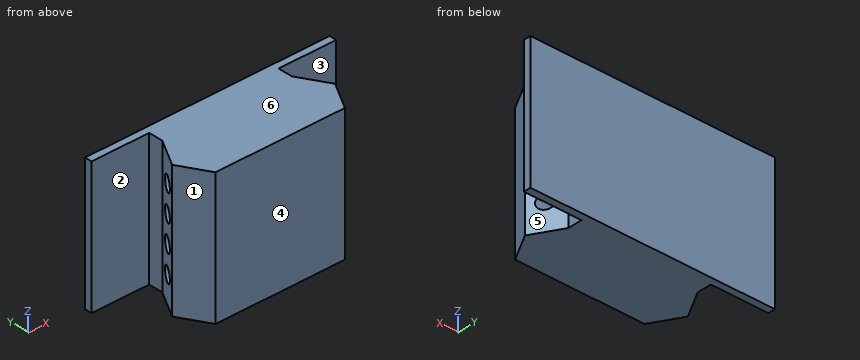
from build123d import *

# Parameters (mm, degrees)
BOSS_EXTRUDE1_DEPTH     = 18.568445
CUT_EXTRUDE1_DEPTH      = 28.942587158
CUT_EXTRUDE1_DEPTH_BACK = 28.942587158
SKETCH2_R               = 1


with BuildPart() as part:
    # Sketch1 → Boss-Extrude1 (new body)
    with BuildSketch(Plane.XY):
        Polygon((9.693000417, 0), (-8.306999583, 0), (-10.641999583, 4.044338636), (-8.306999583, 8.088677271), (-8.306999583, 10.088677271), (-16.306999583, 10.088677271), (-16.306999583, 11.088677271), (17.693000417, 11.088677271), (17.693000417, 10.088677271), (9.693000417, 10.088677271), (9.693000417, 8.088677271), (12.028000417, 4.044338636), align=None)
    extrude(amount=-BOSS_EXTRUDE1_DEPTH)

    # Sketch2 → Cut-Extrude1 (cut, two sides: drawn at the far end of the back side and taken through both)
    with BuildSketch(Plane(origin=(0, 0, 0), x_dir=(0, 0, -1), z_dir=(1, 0, 0)).offset(-CUT_EXTRUDE1_DEPTH_BACK)):
        with Locations(Location((3.71, 5.988677271, 0), (0, 0, 90))):
            Circle(SKETCH2_R)
        with Locations(Location((7.42, 5.988677271, 0), (0, 0, 90))):
            Circle(SKETCH2_R)
        with Locations(Location((11.13, 5.988677271, 0), (0, 0, 90))):
            Circle(SKETCH2_R)
        with Locations(Location((14.84, 5.988677271, 0), (0, 0, 90))):
            Circle(SKETCH2_R)
    extrude(amount=CUT_EXTRUDE1_DEPTH + CUT_EXTRUDE1_DEPTH_BACK, mode=Mode.SUBTRACT)


solid = part.part
Build history of the part. All positions in model axes, mm. Face numbers are marked on the shaded views. A direction names the side the tool comes from. Coordinates: 2 decimals unless noted, no trailing zeros. Order: outer loops, then holes, each group sorted by start corner. A loop starts at its lowest first (then second) coordinate and runs counter-clockwise, first axis right, second up. Notation, with made-up numbers: M 79.25,-39.5 L 137.25,-39.5 A19 ccw 137.25,-31.5 Z; hole C 29,75 d9. An arc over 180 degrees is marked long. One line per question, with ' | ' between items. Start each with the question number.
Q1. Flat gauge pins, fed straight in: pin 1 Ø3 at (y, z) = (5.99, -11.13) entering from -X; pin 2 Ø0.6 at (y, z) = (9.5, -5) entering from -X; pin 3 Ø6.5 at (x, z) = (-13, -10.5) entering from -Y; pin 4 Ø9 at (x, z) = (13.5, -10.5) entering from -Y. Where does each tip first touch, or does it go through?
Q2. 3-axis set-ups, long thin cutter, end or side, ignore diameter. For the marked faces 1 and 2: which of +Z, -Z, +X, -X, +Y, -Y reach the whole face in a straight line?
Q3. Saw through at A-A (y = 6.5). List the corners of the cut face in (x, z), then the cut area to 3 significant figures.
Q4. Saw through at D-D (x = -12.5). List the corners of the cut face in (y, z), then the cut area to 3 significant figures.
Q5. Probe L1, parallel to Y at x = 3, z = -11.13; L2, parallel to Z at x = 10, y = 5.25; L3, parallel to Z at x = -7, y = 5.5. List the from-to ranges inside material, lowest first. Write a range as from..to.
Q6. Saw through at B-B (x = -2). List the corners of the cut face in (y, z).
Q7. Two-plate mould, pull along Y, no slides. Class the marked faces 3, 4, 5 and 6: +Y half, -Y half, draft (parallel to the pull), parting line (faces both ways), or undercut.
Q8. Saw through at C-C (z = -7.42). List the corners of the cut face in (x, y).
Check values:
1) pin 1: stops at x = -10.38 | pin 2: stops at x = -8.31 | pin 3: stops at y = 2.5 | pin 4: stops at y = 0
2) face 1: +Z, -Z, -X, -Y | face 2: +Z, -Z, -X
3) outline: M -9.22,-18.57 L 10.61,-18.57 L 10.61,-15.7 L -9.22,-15.7 Z; M -9.22,-13.98 L 10.61,-13.98 L 10.61,-11.99 L -9.22,-11.99 Z; M -9.22,-10.27 L 10.61,-10.27 L 10.61,-8.28 L -9.22,-8.28 Z; M -9.22,-6.56 L 10.61,-6.56 L 10.61,-4.57 L -9.22,-4.57 Z; M -9.22,-2.85 L 10.61,-2.85 L 10.61,0 L -9.22,0 Z | area: 232 mm2
4) outline: M 10.09,-18.57 L 11.09,-18.57 L 11.09,0 L 10.09,0 Z | area: 18.6 mm2
5) L1: y = 0..4.99, 6.99..11.09 | L2: z = -18.57..-15.51, -14.17..-11.8, -10.46..-8.09, -6.75..-4.38, -3.04..0 | L3: z = -18.57..-15.71, -13.97..-12, -10.26..-8.29, -6.55..-4.58, -2.84..0
6) outline: M 0,-18.57 L 11.09,-18.57 L 11.09,0 L 0,0 Z; hole C 5.99,-14.84 d2; hole C 5.99,-11.13 d2; hole C 5.99,-7.42 d2; hole C 5.99,-3.71 d2
7) face 3: undercut | face 4: -Y half | face 5: undercut | face 6: draft
8) outline: M -16.31,10.09 L -8.31,10.09 L -8.31,8.09 L -8.94,6.99 L 10.33,6.99 L 9.69,8.09 L 9.69,10.09 L 17.69,10.09 L 17.69,11.09 L -16.31,11.09 Z; M -10.64,4.04 L -8.31,0 L 9.69,0 L 12.03,4.04 L 11.48,4.99 L -10.1,4.99 Z
